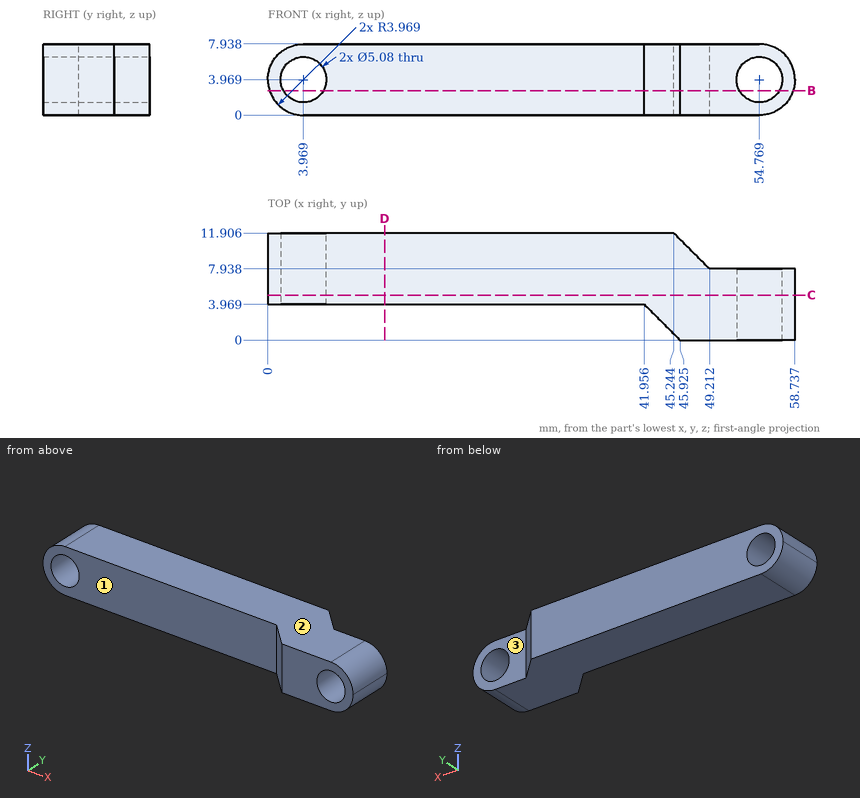
The drawing under review shows one solid part. Ordinate dimensions are in mm from its lowest x, y, z. A direction names the side the tool comes from. Give positions to 0.01 mm unless a question says otherwise; leave off trailing zeros. Order: outer loops, then holes, each group sorted by start corner. A loop starts at its lowest first (then second) coordinate and runs counter-clockwise, first axis right, second up. Notation, with made-up numbers: (-7, -10.75) -> (2, -10.75) arc R22 ccw to (2, 10.25) -> close; hole circle Ø9 at (-17.5, -28.75). An arc over 180 degrees is marked (long way). Write item = value, one per line.
1) For the marked faces 1, 2 and 3, list the 3-axis set-ups (+Z, -Z, +X, -X, +Y, -Y) from which the entire face can be reached by the end or side of a thin tool; tool diameter is ignored.
Findings:
face_1 = +Z, -Z, -X, -Y
face_2 = +Z, +X, -X, +Y, -Y
face_3 = +Z, -Z, +X, +Y
2) We need section C-C, the plane y = 5. Count the separate pieces of the cut face and the enclosed holes in it, and give its area (3 significant figures).
Findings:
separate_pieces = 1
enclosed_holes = 2
area = 412 mm^2
3) We need section B-B, the plane z = 2.75. Give the boundary of the cut face in (x, y) (1 decimal).
Findings:
outline = (0.2, 4) -> (1.7, 4) -> (1.7, 11.9) -> (0.2, 11.9) -> close; (6.2, 4) -> (42, 4) -> (45.9, 0) -> (52.5, 0) -> (52.5, 7.9) -> (49.2, 7.9) -> (45.2, 11.9) -> (6.2, 11.9) -> close; (57, 0) -> (58.5, 0) -> (58.5, 7.9) -> (57, 7.9) -> close
4) To check wall thickness, follow L1, parallel to X at y = 4.25, z = 4; L2, parallel to Z at x = 55, y = 1; L3, parallel to Y at x = 51, z = 4. State the ranges of each line that lie inside material, in increasing order. Write a range as from..to.
Findings:
L1 = 0..1.43, 6.51..52.23, 57.31..58.74
L2 = 0.01..1.44, 6.5..7.93
L3 = 0..7.94
5) Insertion check: pin 1 (2.5 mm diameter, centred on x = 11, z = 4, fed in from -Y); pin 2 (2 mm diameter, centred on y = 3.5, z = 2, fed in from +X). Each pin has a flat end and moves straight along its axis. Give the tip position at first contact, or say it passes through.
Findings:
pin_1 = 3.97
pin_2 = 58.62
6) We need section D-D, the plane x = 13. Give the boundary of the cut face in (y, z), and give its area (3 significant figures).
Findings:
outline = (3.97, 0) -> (11.91, 0) -> (11.91, 7.94) -> (3.97, 7.94) -> close
area = 63.0 mm^2
